CAD build for the part. Positions are in the model's coordinates, mm. A direction names the side the tool comes from. Round coordinates to 2 decimals unless told otherwise and drop trailing zeros. Loops run counter-clockwise (first coordinate to the right, second up) from the corner with the lowest first, then second, coordinate; pieces in that order, holes last. Notation, with made-up numbers: (14, 38) - (50, 38) arc R22 cw to (50, 66) - close; hole circle Ø9 at (48.25, 2.5). An arc over 180 degrees is marked (long way). One line per question, with ' | ' between items.
```python
from build123d import *

# Parameters (mm, degrees)
F0_W            = 55
F0_H            = 46
F0_W_2          = 36
F0_H_2          = 36
F1_DEPTH        = 4
F2_DEPTH        = 10
F3_D            = 5
F3_DEPTH        = 38
F8_D            = 9
F8_DEPTH        = 1
F9_D            = 5
F9_DEPTH        = 13
F9_CSINK_D      = 9
F9_CSINK_ANGLE  = 90
F10_D           = 3
F10_DEPTH       = 38
F10_CSINK_D     = 5
F10_CSINK_ANGLE = 90
F11_R           = 5


with BuildPart() as f1:
    # F0 (on Front) → F1 (new body)
    with BuildSketch(Plane.XZ):
        Rectangle(F0_W, F0_H)
        Rectangle(F0_W_2, F0_H_2, mode=Mode.SUBTRACT)
        Rectangle(F0_W_2, F0_H_2)
    extrude(amount=F1_DEPTH)

    # F0 (on Front) → F2 (join)
    with BuildSketch(Plane.XZ):
        Rectangle(F0_W_2, F0_H_2)
    extrude(amount=-F2_DEPTH)

    # F3
    with Locations(Plane.XZ):
        with Locations((0, 0)):
            Hole(F3_D / 2, depth=F3_DEPTH)

    # F8
    with Locations(Plane.XZ.offset(4)):
        with Locations((0, 0)):
            Hole(F8_D / 2, depth=F8_DEPTH)

    # F9
    with Locations(Plane.XZ.offset(3)):
        with Locations((0, 0)):
            CounterSinkHole(F9_D / 2, F9_CSINK_D / 2, depth=F9_DEPTH, counter_sink_angle=F9_CSINK_ANGLE)

    # F10
    with Locations(Plane(origin=(0, 0, 0), x_dir=(1, 0, 0), z_dir=(0, 1, 0))):
        with Locations((-23.012306, -19.246656), (23.012306, -19.246656), (23.012306, 19.246656), (-23.012306, 19.246656)):
            CounterSinkHole(F10_D / 2, F10_CSINK_D / 2, depth=F10_DEPTH, counter_sink_angle=F10_CSINK_ANGLE)

    # F11
    f11_edges = [f1.edges().sort_by_distance(p)[0] for p in [
        (-27.5, -2, 23),
        (27.5, -2, 23),
        (-27.5, -2, -23),
        (27.5, -2, -23),
    ]]
    fillet(f11_edges, radius=F11_R)


solid = f1.part
```
(1) Tool access for faces 1 (the face through (0, 5, 18)), 2 (the face through (0.59, -3.49, 4.46)), 3 (the face through (0, 5, -18)): list every direction of +Z, -Z, +X, -X, +Y, -Y with a clear straight run to the whole face (end or side of a thin tool).
Results found:
face 1: +Z, +X, -X, +Y | face 2: -Y | face 3: -Z, +X, -X, +Y
(2) Cut at C-C, the plane y = 2.75. Write the cut outline in (x, z).
Results found:
outline: (-18, -18) - (18, -18) - (18, 18) - (-18, 18) - close; hole circle Ø5 at (0, 0)
(3) Cut at A-A, the plane x = 0. Write the cut outline in (y, z), then the cut area to 3 significant figures.
Results found:
outline: (-4, -23) - (0, -23) - (0, -18) - (10, -18) - (10, -2.5) - (-1, -2.5) - (-3, -4.5) - (-4, -4.5) - close; (-4, 4.5) - (-3, 4.5) - (-1, 2.5) - (10, 2.5) - (10, 18) - (0, 18) - (0, 23) - (-4, 23) - close | area: 466 mm²
(4) Drop flat-ended pins along their axis: P1, Ø2.5, axis at x = 23.01, z = -19.25, coming from the -Y side; P2, Ø4, axis at x = -23.01, z = -19.25, coming from the +Y side; P3, Ø5, axis at x = 3, y = 5.5, coming from the +Z side; P4, Ø3, axis at y = 3, z = -2, coming from the +X side. Give the stop position or say it passes through.
Results found:
P1: passes through | P2: stops at y = -0.5 | P3: stops at z = 18 | P4: stops at x = 18
(5) Probe L1, parallel to X at y = 6, z = 0; L2, parallel to Y at x = 20, z = -3.5; L3, parallel to X at y = 4, z = 13.5. List the from-to ranges inside material, lowest first.
Results found:
L1: x = -18 to -2.5, 2.5 to 18 | L2: y = -4 to 0 | L3: x = -18 to 18
(6) Two-plate mould, pull along Z, no slides. Class faces 4 (the face through (-26.07, -2.03, -21.5)), 5 (the face through (-19, 0, 0)), 6 (the face through (26.07, -2.03, 21.5)), 7 (the face through (24.51, -2.52, 19.18)): released by +Z, released by -Z, zero draft, split by the parting line, or undercut.
Results found:
face 4: released by -Z | face 5: zero draft | face 6: released by +Z | face 7: undercut
(7) Cut at B-B, the plane z = 0. Write the cut outline in (x, y).
Results found:
outline: (-27.5, -4) - (-4.5, -4) - (-4.5, -3) - (-2.5, -1) - (-2.5, 10) - (-18, 10) - (-18, 0) - (-27.5, 0) - close; (2.5, -1) - (4.5, -3) - (4.5, -4) - (27.5, -4) - (27.5, 0) - (18, 0) - (18, 10) - (2.5, 10) - close
(8) Cut at D-D, the plane z = 14.5. Write the cut outline in (x, y).
Results found:
outline: (-27.5, -4) - (27.5, -4) - (27.5, 0) - (18, 0) - (18, 10) - (-18, 10) - (-18, 0) - (-27.5, 0) - close
